The figure shows three views and two pictorial views of one solid part (mm, origin at its lowest corner). Answer the questions. A direction names the side the tool comes from. Coordinates: 2 decimals unless noted, no trailing zeros. Order: outer loops, then holes, each group sorted by start corner. A loop starts at its lowest first (then second) coordinate and runs counter-clockwise, first axis right, second up. Notation, with made-up numbers: (-35, -13) - (-18, -13) arc R28 cw to (-18, 11) - close; hole circle Ø6 at (11, 68). An arc over 180 degrees is marked (long way). Use one line per item in the form item = value.
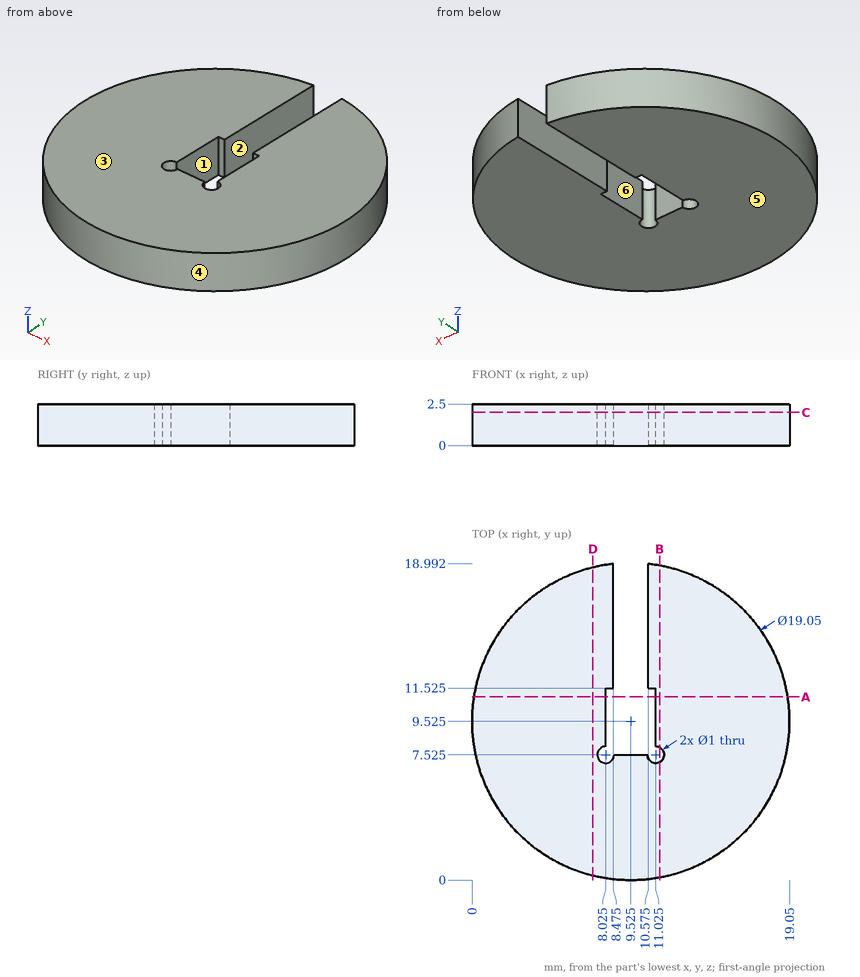
(1) Section B-B, the plane x = 11.25 is taken. Write down the section's boundary in (y, z).
Answer list:
outline = (0.16, 0) - (7.08, 0) - (7.08, 2.5) - (0.16, 2.5) - close; (7.97, 0) - (18.89, 0) - (18.89, 2.5) - (7.97, 2.5) - close
(2) The mould has two halves that part along Y. Classify the marked faces 4, 5 and 6: +Y half, -Y half, draft (parallel to the pull), parting line (faces both ways), or undercut.
Answer list:
face_4 = parting line
face_5 = draft
face_6 = undercut
(3) Given pin 1 Ø1 at (y, z) = (12, 0.5) entering from +X; pin 2 Ø1 at (y, z) = (16, 1.5) entering from +X, each flat-ended and moving along its own axis, determine where each tip first touches the part or whether it passes through.
Answer list:
pin_1 = 18.84
pin_2 = 16.94
(4) Straight lines are drawn through the part: L1, parallel to X at y = 10, z = 1.95 (3 decimals); L2, parallel to X at y = 18, z = 0.6 (1 decimal); L3, parallel to Y at x = 10.75, z = 1.35 (1 decimal). For each, find the intervals that lie inside material, in ascending order.
Answer list:
L1 = 0.012 to 8.025, 11.025 to 19.038
L2 = 5.2 to 8.5, 10.6 to 13.9
L3 = 0.1 to 7.1, 11.5 to 19
(5) Which of the six approach directions +Z, -Z, +X, -X, +Y, -Y give full straight-line access (tool end or side, diameter ignored) to the marked faces 1, 2 and 3?
Answer list:
face_1 = +Z, -Z
face_2 = +Z, -Z, +Y
face_3 = +Z, +X, -X, +Y, -Y
(6) Section D-D, the plane x = 7.25 is taken. Write down the section's boundary in (y, z).
Answer list:
outline = (0.28, 0) - (18.77, 0) - (18.77, 2.5) - (0.28, 2.5) - close
(7) Section A-A, the plane y = 11 is taken. Write down the section's boundary in (x, z) (3 decimals).
Answer list:
outline = (0.115, 0) - (8.025, 0) - (8.025, 2.5) - (0.115, 2.5) - close; (11.025, 0) - (18.935, 0) - (18.935, 2.5) - (11.025, 2.5) - close
(8) Section C-C, the plane z = 2 is taken. Write down the section's boundary in (x, y) (3 decimals), then the cut area to 3 significant figures.
Answer list:
outline = (8.025, 8.025) - (8.025, 11.525) - (8.475, 11.525) - (8.475, 18.992) arc R9.525 ccw (long way) to (10.575, 18.992) - (10.575, 11.525) - (11.025, 11.525) - (11.025, 8.025) arc R0.5 cw (long way) to (10.525, 7.525) - (8.525, 7.525) arc R0.5 cw (long way) to start
area = 256 mm2
